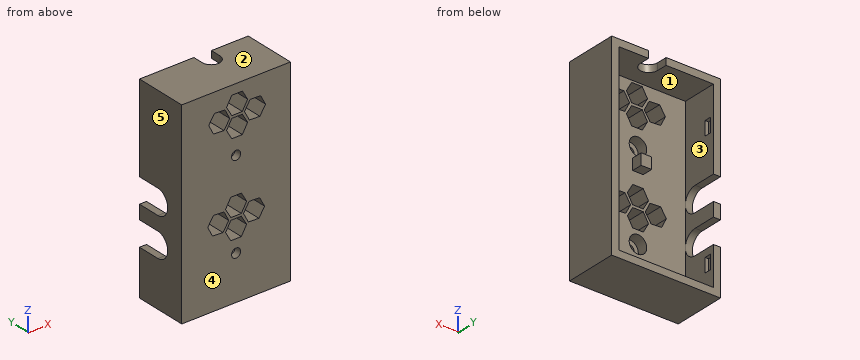
```python
from build123d import *

# Parameters (mm, degrees)
ESQUISSE1_W             = 31
ESQUISSE1_H             = 56
BOSS_EXTRU_1_DEPTH      = 5
ESQUISSE2_R             = 1.3
ENL_V_MAT_EXTRU_1_DEPTH = 65.202803677
ESQUISSE4_R             = 2.5
ENL_V_MAT_EXTRU_2_DEPTH = 3
ESQUISSE5_W             = 3
ESQUISSE5_H             = 3
ESQUISSE5_H_2           = 3.199702253
BOSS_EXTRU_2_DEPTH      = 3
ESQUISSE6_W             = 31
ESQUISSE6_H             = 56
ESQUISSE6_W_2           = 27
ESQUISSE6_H_2           = 52
BOSS_EXTRU_3_DEPTH      = 10
ENL_V_MAT_EXTRU_3_DEPTH = 10
ENL_V_MAT_EXTRU_4_DEPTH = 10
ESQUISSE10_W            = 4
ESQUISSE10_H            = 2
ENL_V_MAT_EXTRU_5_DEPTH = 1
ESQUISSE11_W            = 4
ESQUISSE11_H            = 2
ENL_V_MAT_EXTRU_6_DEPTH = 1


with BuildPart() as part:
    # Esquisse1 → Boss.-Extru.1 (new body)
    with BuildSketch(Plane(origin=(0, 0, 0), x_dir=(1, 0, 0), z_dir=(0, 1, 0))):
        with Locations((15.5, 28)):
            Rectangle(ESQUISSE1_W, ESQUISSE1_H)
    extrude(amount=BOSS_EXTRU_1_DEPTH)

    # Esquisse2 → Enlèv. mat.-Extru.1 (cut, through all)
    with BuildSketch(Plane(origin=(0, 5, 0), x_dir=(1, 0, 0), z_dir=(0, 1, 0))):
        with Locations(Location((15.5, 43.356492458, 0), (0, 0, 270))):
            Circle(ESQUISSE2_R)
        with Locations(Location((15.5, 18.356492458, 0), (0, 0, 270))):
            Circle(ESQUISSE2_R)
        Polygon((13.411017957, 34.281896818), (11.768091764, 36.801158467), (8.764884081, 36.637973473), (7.40460259, 33.955526829), (9.047528783, 31.43626518), (12.050736466, 31.599450174), align=None)
        Polygon((18.507637899, 37.071867086), (17.003818949, 39.676557912), (13.996181051, 39.676557912), (12.492362101, 37.071867086), (13.996181051, 34.46717626), (17.003818949, 34.46717626), align=None)
        Polygon((18.507637899, 31.162485434), (17.003818949, 33.76717626), (13.996181051, 33.76717626), (12.492362101, 31.162485434), (13.996181051, 28.557794609), (17.003818949, 28.557794609), align=None)
        Polygon((23.612406723, 34.235887688), (22.008252208, 36.780013083), (19.002897728, 36.662837218), (17.601697764, 34.001535959), (19.205852279, 31.457410565), (22.211206759, 31.574586429), align=None)
        Polygon((13.692694357, 8.311332727), (12.049768165, 10.830594377), (9.046560481, 10.667409382), (7.68627899, 7.984962739), (9.329205183, 5.465701089), (12.332412866, 5.628886084), align=None)
        Polygon((18.789314299, 11.101302996), (17.28549535, 13.705993821), (14.277857451, 13.705993821), (12.774038501, 11.101302996), (14.277857451, 8.49661217), (17.28549535, 8.49661217), align=None)
        Polygon((18.789314299, 5.191921344), (17.28549535, 7.79661217), (14.277857451, 7.79661217), (12.774038501, 5.191921344), (14.277857451, 2.587230518), (17.28549535, 2.587230518), align=None)
        Polygon((23.894083123, 8.265323598), (22.289928608, 10.809448992), (19.284574129, 10.692273128), (17.883374164, 8.030971869), (19.487528679, 5.486846474), (22.492883159, 5.604022339), align=None)
    extrude(amount=-ENL_V_MAT_EXTRU_1_DEPTH, mode=Mode.SUBTRACT)

    # Esquisse4 → Enlèv. mat.-Extru.2 (cut)
    with BuildSketch(Plane(origin=(0, 5, 0), x_dir=(1, 0, 0), z_dir=(0, 1, 0))):
        with Locations(Location((15.5, 43.356492458, 0), (0, 0, 270))):
            Circle(ESQUISSE4_R)
        with Locations(Location((15.5, 18.356492458, 0), (0, 0, 270))):
            Circle(ESQUISSE4_R)
    extrude(amount=-ENL_V_MAT_EXTRU_2_DEPTH, mode=Mode.SUBTRACT)

    # Esquisse5 → Boss.-Extru.2 (add)
    with BuildSketch(Plane(origin=(0, 5, 0), x_dir=(1, 0, 0), z_dir=(0, 1, 0))):
        with Locations((15.5, 52.5)):
            Rectangle(ESQUISSE5_W, ESQUISSE5_H)
        with Locations((15.5, 23.400148874)):
            Rectangle(ESQUISSE5_W, ESQUISSE5_H_2)
    extrude(amount=BOSS_EXTRU_2_DEPTH)

    # Esquisse6 → Boss.-Extru.3 (add)
    with BuildSketch(Plane(origin=(0, 5, 0), x_dir=(1, 0, 0), z_dir=(0, 1, 0))):
        with Locations((15.5, 28)):
            Rectangle(ESQUISSE6_W, ESQUISSE6_H)
        with Locations((15.5, 28)):
            Rectangle(ESQUISSE6_W_2, ESQUISSE6_H_2, mode=Mode.SUBTRACT)
    extrude(amount=BOSS_EXTRU_3_DEPTH)

    # Esquisse8 → Enlèv. mat.-Extru.3 (cut)
    with BuildSketch(Plane.ZY):
        with BuildLine():
            Line((-43, 15), (-43, 8.5))
            ThreePointArc((-43, 8.5), (-39.5, 5), (-36, 8.5))
            Line((-36, 8.5), (-36, 15))
            Line((-36, 15), (-43, 15))
        make_face()
        with BuildLine():
            Line((-32, 15), (-32, 8.5))
            ThreePointArc((-32, 8.5), (-28.5, 5), (-25, 8.5))
            Line((-25, 8.5), (-25, 15))
            Line((-25, 15), (-32, 15))
        make_face()
    extrude(amount=-ENL_V_MAT_EXTRU_3_DEPTH, mode=Mode.SUBTRACT)

    # Esquisse9 → Enlèv. mat.-Extru.4 (cut)
    with BuildSketch(Plane.XY):
        with BuildLine():
            Line((15.5, 15), (15.5, 12))
            ThreePointArc((15.5, 12), (18, 9.5), (20.5, 12))
            Line((20.5, 12), (20.5, 15))
            Line((20.5, 15), (15.5, 15))
        make_face()
    extrude(amount=-ENL_V_MAT_EXTRU_4_DEPTH, mode=Mode.SUBTRACT)

    # Esquisse10 → Enlèv. mat.-Extru.5 (cut)
    with BuildSketch(Plane.ZY.offset(-29)):
        with Locations((-43, 13)):
            Rectangle(ESQUISSE10_W, ESQUISSE10_H)
        with Locations((-14, 13)):
            Rectangle(ESQUISSE10_W, ESQUISSE10_H)
    extrude(amount=-ENL_V_MAT_EXTRU_5_DEPTH, mode=Mode.SUBTRACT)

    # Esquisse11 → Enlèv. mat.-Extru.6 (cut)
    with BuildSketch(Plane(origin=(2, 0, 0), x_dir=(0, 0, -1), z_dir=(1, 0, 0))):
        with Locations((12, 13)):
            Rectangle(ESQUISSE11_W, ESQUISSE11_H)
        with Locations((47, 13)):
            Rectangle(ESQUISSE11_W, ESQUISSE11_H)
    extrude(amount=-ENL_V_MAT_EXTRU_6_DEPTH, mode=Mode.SUBTRACT)


solid = part.part
```
The model under review builds one solid part; all positions refer to its coordinate system, in mm. Face numbers are marked on the shaded views. A direction names the side the tool comes from. Round coordinates to 2 decimals unless told otherwise and drop trailing zeros. Loops run counter-clockwise (first coordinate to the right, second up) from the corner with the lowest first, then second, coordinate; pieces in that order, holes last. Notation, with made-up numbers: M 59,-0.75 L 97,-0.75 A26 cw 97,33.25 Z; hole C 77.25,88 d5. An arc over 180 degrees is marked long. Write item = value, one per line.
Item 1: Take a section at D-D on y = 13.25. State how many separate pieces and enclosed holes the cut face has, then the cut area to 3 significant figures.
Return value:
separate_pieces = 3
enclosed_holes = 0
area = 278 mm2
Item 2: Machinability: for the marked faces 1 and 2, which of the approach directions +Z, -Z, +X, -X, +Y, -Y give a long, thin tool a straight path to every point of the face, cutting with its end or side? Answer none if there is none.
Return value:
face_1 = +Y
face_2 = +Z, +X, -X, +Y, -Y
Item 3: Take a section at C-C on z = -7. Write out the cut boundary in (x, y).
Return value:
outline = M 0,0 L 8.33,0 L 8.33,5 L 2,5 L 2,15 L 0,15 Z; M 13.03,0 L 13.82,0 L 13.82,5 L 13.03,5 Z; M 17.75,0 L 18.53,0 L 18.53,5 L 17.75,5 Z; M 23.23,0 L 31,0 L 31,15 L 29,15 L 29,5 L 23.23,5 Z
Item 4: For line 1 (Z direction, x = 16, y = 10); line 2 (X direction, y = 4.75, z = -33); line 3 (X direction, y = 7, z = -49), list the stretches that pass through material, from the lowest coordinate up. Write a range as [from, to].
Return value:
line_1 = [-56, -54], [-2, 0]
line_2 = [0, 8.03], [12.76, 13.55], [17.45, 18.23], [22.96, 31]
line_3 = [0, 2], [29, 31]
Item 5: Take a section at B-B on x = 4. Write out the cut boundary in (y, z).
Return value:
outline = M 0,-56 L 15,-56 L 15,-54 L 5,-54 L 5,-2 L 15,-2 L 15,0 L 0,0 Z
Item 6: Insertion check: P1, Ø1.5, axis at y = 10, z = -40.5, coming from the -X side; P2, Ø5.5, axis at x = 16, z = -44.5, coming from the +Y side; P3, Ø3, axis at x = 21.5, z = -34.5, coming from the +Y side. Each pin has a flat end and moves straight along its axis. Give the tip position at first contact, or say it passes through.
Return value:
P1 = 29
P2 = 5
P3 = through
Item 7: Take a section at A-A on z = -38.5. Write out the cut boundary in (x, y), then the cut area to 3 significant figures.
Return value:
outline = M 0,0 L 13.32,0 L 13.32,5 L 2,5 L 2,5.15 L 0,5.15 Z; M 17.68,0 L 31,0 L 31,15 L 29,15 L 29,5 L 17.68,5 Z
area = 153 mm2
Item 8: The part is to be moulded in two halves that separate along X. For the marked faces 3, 4 and 5, say which applies: released by +X, released by -X, zero draft, split by the parting line, or undercut.
Return value:
face_3 = undercut
face_4 = zero draft
face_5 = released by -X
